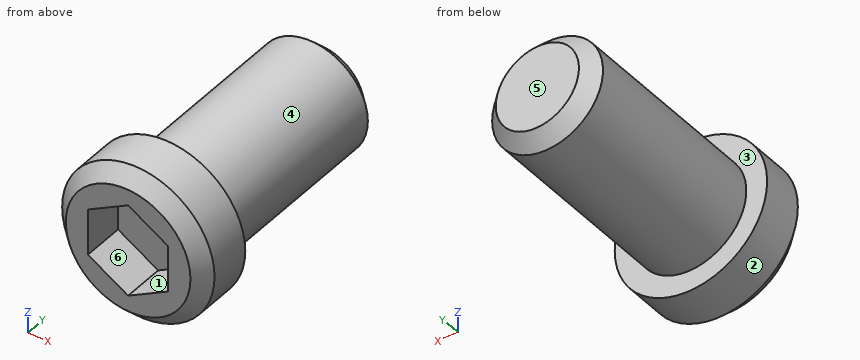
Solid Edge part; units mm, degrees
sketch "Sketch1" plane through (0, 0, 0) normal (0, -1, 0) x (1, 0, 0)
  circle A0 centre (0, 0) radius 4
extrude "Protrusion1" add sketch "Sketch1" against normal blind 15
sketch "Sketch2" plane through (0, 0, 0) normal (0, -1, 0) x (1, 0, 0)
  circle A0 centre (0, 0) radius 5.5
extrude "ProtrusiónExtruida_2" add sketch "Sketch2" along normal blind 4
chamfer "Chaflán_1" distance 1 angle 45 1 edges at (-5.5, -4, 0)
sketch "Sketch3" plane through (0, -4, 0) normal (0, -1, 0) x (0, 0, 1)
  line L0 (1.6725, -2.8968) -> (3.3449, 0)
  line L1 (3.3449, 0) -> (1.6725, 2.8968)
  line L2 (1.6725, 2.8968) -> (-1.6725, 2.8968)
  line L3 (-1.6725, 2.8968) -> (-3.3449, 0)
  line L4 (-3.3449, 0) -> (-1.6725, -2.8968)
  line L5 (-1.6725, -2.8968) -> (1.6725, -2.8968)
extrude "VaciadoExtruido_1" cut sketch "Sketch3" against normal blind 2.9342
chamfer "Chaflán_4" distance 1 angle 45 1 edges at (-4, 15, 0)
properties material "Steel - Structural:1.0035 , S185"
Can you work these out from the model? Positions are in its coordinate system, mm. Face numbers are marked on the shaded views. A direction names the side the tool comes from. Coordinates: 2 decimals unless noted, no trailing zeros. Loops run counter-clockwise (first coordinate to the right, second up) from the corner with the lowest first, then second, coordinate; pieces in that order, holes last. Notation, with made-up numbers: (29, 18.25) -> (57, 18.25) arc R24 ccw to (57, 47.25) -> close; hole circle Ø8 at (-23.5, 80). An arc over 180 degrees is marked (long way). Answer as a JSON object with one key per item and string values.
1) For the marked faces 1, 2 and 3, which set-ups out of +Z, -Z, +X, -X, +Y, -Y let a thin tool reach every point of the face, with its end or its side?
Results:
{"face 1": "-Y", "face 2": "+Y, -Y", "face 3": "+Y"}
2) Imagine slicing it at A-A (y = -2.25). Please give me the cut outline in (x, z), then the cut area to 3 significant figures.
Results:
{"outline": "circle Ø11 at (0, 0); hole (-2.9, -1.67) -> (0, -3.34) -> (2.9, -1.67) -> (2.9, 1.67) -> (0, 3.34) -> (-2.9, 1.67) -> close", "area": "66.0 mm^2"}
3) If I drill on line 1 (Z direction, x = 1.5, y = -1.25); line 2 (Y direction, x = 1.5, z = -1.5); line 3 (Y direction, x = -3.75, z = -1), over which ranges is the centre line in solid material (lowest first)?
Results:
{"line 1": "z = -5.29 to -2.48, 2.48 to 5.29", "line 2": "y = -1.07 to 15", "line 3": "y = -4 to 14.12"}
4) For P1, Ø6, axis at y = 6, z = 4, coming from the -X side; P2, Ø1.7, axis at x = 1, z = 1, coming from the -Y side; P3, Ø4, axis at x = -4, z = -3.5, coming from the +Y side, each with a flat end and sliding along its axis, tell me the tip position at first contact or that it passes through.
Results:
{"P1": "stops at x = -3.87", "P2": "stops at y = -1.07", "P3": "stops at y = 14.68"}
5) Thinking about a two-plate mould opening in Z: for the marked faces 4, 5 and 6, which applies, pulls with the +Z half, pulls with the -Z half, needs draft (parallel to the pull), parting line crosses it, or undercut?
Results:
{"face 4": "parting line crosses it", "face 5": "needs draft", "face 6": "undercut"}
6) Imagine slicing it at B-B (z = 0). Please give me the cut outline in (x, y), then the cut area to 3 significant figures.
Results:
{"outline": "(-5.5, -3) -> (-4.5, -4) -> (-2.9, -4) -> (-2.9, -1.07) -> (2.9, -1.07) -> (2.9, -4) -> (4.5, -4) -> (5.5, -3) -> (5.5, 0) -> (4, 0) -> (4, 14) -> (3, 15) -> (-3, 15) -> (-4, 14) -> (-4, 0) -> (-5.5, 0) -> close", "area": "145 mm^2"}
7) Imagine slicing it at C-C (y = 2.5). Please give me the cut outline in (x, z).
Results:
{"outline": "circle Ø8 at (0, 0)"}
